Model file for the job. Use its own axes, mm. A direction names the side the tool comes from. Give positions to 0.01 mm unless a question says otherwise; leave off trailing zeros. Write each loop counter-clockwise with the first axis right and the second up, starting at its lowest first coordinate (ties: lowest second). Pieces come first, ordered by that corner, then holes. Notation, with made-up numbers: (56.5, 79) - (110.5, 79) arc R21 cw to (110.5, 105) - close; hole circle Ø4 at (22, 59). An arc over 180 degrees is marked (long way). One line per item, written item: value. Start each with the question number.
(1) Drop a flat-ended pin along its axis: P1, Ø10, axis at y = -9.5, z = -13.5, coming from the +X side. Give the stop position or say it passes through.
(2) Probe L1, parallel to Y at x = 12.5, z = -8.5; L2, parallel to Y at x = 12.25, z = 15; L3, parallel to Z at x = 4, y = -22.5. List the from-to ranges inside material, lowest first.
(3) Cut at C-C, the plane z = 26. List the corners of the cut face in (x, y), and give its area (3 significant figures).
(4) Cut at B-B, the plane x = 1. State how many separate pieces and enclosed holes the cut face has, and give its area (3 significant figures).
(5) Mould opens along Z. For faces 3 (the face through (8.45, -19.27, 28.25)), 4 (the face through (16.668, 0, -20)), 5 (the face through (8.217, 23.111, -12.427)) say: pulls with the +Z half, pulls with the -Z half, needs draft (parallel to the pull), parting line crosses it, or undercut.
(6) Cut at A-A, the plane z = 14.5. List the corners of the cut face in (x, y), and give its area (3 significant figures).
(7) Cut at D-D, the plane y = -16. List the corners of the cut face in (x, z).
(8) 3-axis set-ups, long thin cutter, end or side, ignore diameter. For faces 1 (the face through (8, 17.462, 12)), 2 (the face through (8.217, -21.999, -12.023)): which of +Z, -Z, +X, -X, +Y, -Y reach the whole face in a straight line?
Autodesk Inventor part; units mm, degrees
ref_plane "YZ Plane" through (0, 0, 0) normal (1, 0, 0) x (0, 1, 0)
ref_plane "XZ Plane" through (0, 0, 0) normal (0, 1, 0) x (-1, 0, 0)
ref_plane "XY Plane" through (0, 0, 0) normal (0, 0, 1) x (1, 0, 0)
sketch "Sketch2" plane through (0, 0, 0) normal (1, 0, 0) x (0, 1, 0)
  line L0 (30.1625, 30.1625) -> (30.1625, -30.1625)
  line L1 (30.1625, -30.1625) -> (-30.1625, -30.1625)
  line L2 (-30.1625, -30.1625) -> (-30.1625, 30.1625)
  line L3 (-30.1625, 30.1625) -> (30.1625, -30.1625) construction
  line L4 (30.1625, 30.1625) -> (-30.1625, -30.1625) construction
  arc A0 (-17.4625, 0) -> (17.4625, 0) centre (0, 0) ccw
  circle A1 centre (-23.4665, 9.7202) radius 2.7305
  circle A2 centre (-23.4665, -9.7202) radius 2.7305
  circle A3 centre (-9.7202, -23.4665) radius 2.7305
  circle A4 centre (9.7202, -23.4665) radius 2.7305
  circle A5 centre (23.4665, -9.7202) radius 2.7305
  circle A6 centre (23.4665, 9.7202) radius 2.7305
  circle A7 centre (9.7202, 23.4665) radius 2.7305
  circle A8 centre (-9.7202, 23.4665) radius 2.7305
  line L5 (-17.4625, 0) -> (-17.4625, 30.1625)
  line L6 (17.4625, 0) -> (17.4625, 30.1625)
  line L7 (-30.1625, 30.1625) -> (-17.4625, 30.1625)
  line L8 (17.4625, 30.1625) -> (30.1625, 30.1625)
  dimension "d14" = 25.4
  dimension "d19" = 34.925
  dimension "d20" = 60.325
  dimension "d21" = 5.461
  dimension "d24" = 360
extrude "Extrusion1" add sketch "Sketch2" along normal blind 16.6675 contours L0 L1 L2 L7 L5 A0 L6 L8 | A3 | A4
fillet "Fillet1" radius 6.35 6 edges at (8.3337, 30.1625, -30.1625) (8.3337, 30.1625, 30.1625) (8.3337, 17.4625, 30.1625) (8.3337, -17.4625, 30.1625) (8.3337, -30.1625, 30.1625) (8.3337, -30.1625, -30.1625)
properties part number "3DPRINT,KICKER,MOTOR,MOUNT" material "Nylon 6/6"
Answers follow:
1. P1: stops at x = 16.67
2. L1: y = -30.16 to -25.91, -21.02 to -15.25, 15.25 to 21.02, 25.91 to 30.16
2. L2: y = -30.16 to -17.46, 17.46 to 30.16
2. L3: z = -30.16 to -12.27, -7.17 to 7.17, 12.27 to 30.03
3. outline: (0, -29.77) - (16.67, -29.77) - (16.67, -17.85) - (0, -17.85) - close; (0, 17.85) - (16.67, 17.85) - (16.67, 29.77) - (0, 29.77) - close
3. area: 397 mm²
4. separate pieces: 1
4. enclosed holes: 4
4. area: 1,960 mm²
5. face 3: pulls with the +Z half
5. face 4: needs draft
5. face 5: undercut
6. outline: (0, -30.16) - (16.67, -30.16) - (16.67, -17.46) - (0, -17.46) - close; (0, 17.46) - (16.67, 17.46) - (16.67, 30.16) - (0, 30.16) - close
6. area: 423 mm²
7. outline: (0, -30.16) - (16.67, -30.16) - (16.67, -7) - (0, -7) - close
8. face 1: +Z, +X, -X
8. face 2: +X, -X
